Geometry: final body of the model. Coordinates: model frame, mm. A direction names the side the tool comes from. Round coordinates to 2 decimals unless told otherwise and drop trailing zeros. Write each loop counter-clockwise with the first axis right and the second up, starting at its lowest first coordinate (ties: lowest second). Pieces come first, ordered by that corner, then holes. Notation, with made-up numbers: (-34.5, 80.5) -> (-2.5, 80.5) arc R21 cw to (-2.5, 100.5) -> close; hole circle Ø6 at (-31, 20.25). An arc over 180 degrees is marked (long way). Use one line per item in the form item = value. Start each with the question number.
1. Cut plane B-B, the plane y = 0.5. Return the cut outline in (x, z) (3 decimals).
2. Pin query (flat end, axial travel): pin 1 Ø3 at (y, z) = (14, 27) entering from +X; pin 2 Ø9.5 at (x, z) = (-16.5, 22) entering from -Y; pin 3 Ø4.5 at (x, z) = (16, 25.5) entering from +Y. Return the tip coordinate at first contact, or that it passes through.
3. Cut plane A-A, the plane x = 0. Return the cut outline in (y, z) (3 decimals).
4. Cut plane C-C, the plane z = 22. State how many separate pieces and enclosed holes the cut face has, plus the area to 3 significant figures.
5. Draft query along Y for faces 5 (the face through (15, -23.05, 21)), 6 (the face through (13, 26, 8)), 7 (the face through (0, 12.525, 11)). Return one class per face: pulls with the +Y half, pulls with the -Y half, needs draft (parallel to the pull), parting line crosses it, or undercut.
6. Reachability of faces 1 (the face through (14, -26, 8)), 2 (the face through (-15, -19.05, 21)), 3 (the face through (10.35, 10, 25)), 4 (the face through (0, 27.75, 14)) from +Z, -Z, +X, -X, +Y, -Y: full face, straight path, thin tool, end or side. Return the list, or none.
7. Line query: L1, parallel to Y at x = -4.5, z = 15 (3 decimals); L2, parallel to X at y = 3, z = 6; L3, parallel to Y at x = 12.5, z = 29. Output: solid intervals per line, ascending.
8. Cut plane D-D, the plane x = 5.5. Return the cut outline in (y, z) (3 decimals).
```python
from build123d import *

# Parameters (mm, degrees)
F1_DEPTH  = 31.75
F2_T      = -4
F3_W      = 4
F3_H      = 10
F4_DEPTH  = 63.5
F6_DEPTH  = 8
F8_DEPTH  = 2
F11_DEPTH = 4
F13_DEPTH = 4
F14_W     = 12.7
F14_H     = 4
F15_DEPTH = 10
F16_SIZE  = 5
F17_R     = 2.15
F18_DEPTH = 25
F19_W     = 30.1
F19_H     = 4


# Not quite as in the source:
# - a pattern or mirror of a feature is missing from the dataset's text; its kind, count and spacing are read off the source's solid


with BuildPart() as f1:
    # F0 (on Front) → F1 (new body, symmetric)
    with BuildSketch(Plane.XZ):
        Polygon((-10.35, 0), (10.35, 0), (10.35, 31.575), (6.35, 31.575), (-6.35, 31.575), (-10.35, 31.575), align=None)
    extrude(amount=F1_DEPTH, both=True)

    # F2
    f2_openings = [f1.faces().sort_by_distance(p)[0] for p in [
        (0, 0, 0),
    ]]
    offset(amount=F2_T, openings=f2_openings)

    # F3 (on face) → F4 (join, through all)
    with BuildSketch(Plane.XZ.offset(31.75)):
        with Locations((-8.35, 36.575)):
            Rectangle(F3_W, F3_H)
        with Locations((8.35, 36.575)):
            Rectangle(F3_W, F3_H)
    extrude(amount=-F4_DEPTH)

    # F5 (on Top) → F6 (join)
    with BuildSketch(Plane.XY):
        Polygon((-19.05, -23.05), (-10.35, -31.75), (-10.35, 31.75), (-19.05, 23.05), align=None)
        Polygon((10.35, 31.75), (10.35, -31.75), (19.05, -23.05), (19.05, 23.05), align=None)
    extrude(amount=F6_DEPTH)

    # F7 (on Front) → F8 (join, symmetric)
    with BuildSketch(Plane.XZ):
        Polygon((-19.05, 8), (-10.35, 8), (-10.35, 41.575), (-19.05, 32.875), align=None)
        Polygon((10.35, 8), (19.05, 8), (19.05, 32.875), (10.35, 41.575), align=None)
    f8 = extrude(amount=F8_DEPTH, both=True)

    # F8_copies: F8 across plane
    add(f8.mirror(Plane(origin=(0, -10.525, 0), x_dir=(0, 0, -1), z_dir=(0, -1, 0))))

    # F10 (on plane+point) → F11 (join)
    with BuildSketch(Plane.XZ.offset(-23.05)):
        Polygon((10.35, 8), (19.05, 8), (19.05, 32.875), (10.35, 41.575), align=None)
        Polygon((-19.05, 32.875), (-19.05, 8), (-10.35, 8), (-10.35, 41.575), align=None)
    extrude(amount=F11_DEPTH)

    # F12 (on face) → F13 (cut)
    with BuildSketch(Plane(origin=(0, 0, 0), x_dir=(1, 0, 0), z_dir=(0, 0, -1))):
        Polygon((-8.6931457505, -27.75), (8.6931457505, -27.75), (15.05, -21.3931457505), (15.05, 21.3931457505), (8.6931457505, 27.75), (-8.6931457505, 27.75), (-15.05, 21.3931457505), (-15.05, -21.3931457505), align=None)
    extrude(amount=-F13_DEPTH, mode=Mode.SUBTRACT)

    # F14 (on face) → F15 (join, through all)
    with BuildSketch(Plane.XY.offset(31.575)):
        with Locations((0, 29.75)):
            Rectangle(F14_W, F14_H)
    extrude(amount=F15_DEPTH)

    # F16
    f16_edges = [f1.edges().sort_by_distance(p)[0] for p in [
        (8.35, -31.75, 41.575),
        (-8.35, -31.75, 41.575),
    ]]
    chamfer(f16_edges, length=F16_SIZE)

    # F17 (on face) → F18 (cut)
    with BuildSketch(Plane.XY.offset(31.575)):
        with Locations((0, -10.525)):
            Circle(F17_R)
    extrude(amount=-F18_DEPTH, mode=Mode.SUBTRACT)

    # F19 (on face) → F20 (join, up to the next surface of F1)
    with BuildSketch(Plane(origin=(0, 0, 0), x_dir=(1, 0, 0), z_dir=(0, 0, -1))):
        with Locations((0, -10.525)):
            Rectangle(F19_W, F19_H)
    extrude(until=Until.NEXT, dir=(0, 0, 1))


solid = f1.part
```
Outcome:
q1.outline = (-19.05, 0) -> (-15.05, 0) -> (-15.05, 4) -> (-6.35, 4) -> (-6.35, 27.575) -> (6.35, 27.575) -> (6.35, 4) -> (15.05, 4) -> (15.05, 0) -> (19.05, 0) -> (19.05, 32.875) -> (10.35, 41.575) -> (6.35, 41.575) -> (6.35, 31.575) -> (-6.35, 31.575) -> (-6.35, 41.575) -> (-10.35, 41.575) -> (-19.05, 32.875) -> close
q2.pin_1 = 10.35
q2.pin_2 = -23.05
q2.pin_3 = 23.05
q3.outline = (-31.75, 0) -> (-27.75, 0) -> (-27.75, 27.575) -> (-12.675, 27.575) -> (-12.675, 31.575) -> (-31.75, 31.575) -> close; (-8.375, 27.575) -> (8.525, 27.575) -> (8.525, 0) -> (12.525, 0) -> (12.525, 27.575) -> (27.75, 27.575) -> (27.75, 0) -> (31.75, 0) -> (31.75, 41.575) -> (27.75, 41.575) -> (27.75, 31.575) -> (-8.375, 31.575) -> close
q4.separate_pieces = 1
q4.enclosed_holes = 2
q4.area = 869 mm^2
q5.face_5 = pulls with the -Y half
q5.face_6 = needs draft
q5.face_7 = undercut
q6.face_1 = +Z, +X, -Y
q6.face_2 = +Z, -X
q6.face_3 = +Z, +X
q6.face_4 = -Z
q7.L1 = -31.75 to -27.75, 8.525 to 12.525, 27.75 to 31.75
q7.L2 = -19.05 to -6.35, 6.35 to 19.05
q7.L3 = -23.05 to -19.05, -2 to 2, 19.05 to 23.05
q8.outline = (-31.75, 0) -> (-27.75, 0) -> (-27.75, 27.575) -> (8.525, 27.575) -> (8.525, 0) -> (12.525, 0) -> (12.525, 27.575) -> (27.75, 27.575) -> (27.75, 0) -> (31.75, 0) -> (31.75, 41.575) -> (27.75, 41.575) -> (27.75, 31.575) -> (-31.75, 31.575) -> close
